Check sheet for the modelled part. Datum: model origin and axes. Units: mm. A direction names the side the tool comes from. Round coordinates to 2 decimals unless told otherwise and drop trailing zeros. Write each loop counter-clockwise with the first axis right and the second up, starting at its lowest first coordinate (ties: lowest second). Pieces come first, ordered by that corner, then holes. Notation, with made-up numbers: (-27, 54) -> (2, 54) arc R12 ccw to (2, 72) -> close; hole circle Ø8 at (46, -10.75). An arc over 180 degrees is marked (long way). One line per item, written item: value.
Autodesk Inventor part; units mm, degrees
ref_plane "YZ Plane" through (0, 0, 0) normal (1, 0, 0) x (0, 1, 0)
ref_plane "XZ Plane" through (0, 0, 0) normal (0, 1, 0) x (-1, 0, 0)
ref_plane "XY Plane" through (0, 0, 0) normal (0, 0, 1) x (1, 0, 0)
sketch "Sketch1" plane through (0, 0, 0) normal (0, 1, 0) x (-1, 0, 0)
  line L0 (-19.05, -25.4) -> (19.05, -25.4)
  line L1 (19.05, -25.4) -> (19.05, 25.4)
  line L2 (19.05, 25.4) -> (-19.05, 25.4)
  line L3 (-19.05, 25.4) -> (-19.05, -25.4)
  line L4 (-19.05, -25.4) -> (19.05, 25.4) construction
  line L5 (19.05, -25.4) -> (-19.05, 25.4) construction
  line L6 (-15.875, 22.225) -> (15.875, 22.225)
  line L7 (15.875, 22.225) -> (15.875, -22.225)
  line L8 (15.875, -22.225) -> (-15.875, -22.225)
  line L9 (-15.875, -22.225) -> (-15.875, 22.225)
  point P0 (0, 0)
  dimension "d0" = 38.1
  dimension "d1" = 50.8
  dimension "d2" = 3.175
extrude "Extrusion1" add sketch "Sketch1" along normal blind 508
sketch "Sketch2" plane through (19.05, 0, 25.4) normal (1, 0, 0) x (0, 0, -1)
  line L0 (25.4, 469.9) -> (25.4, 393.7) construction
  line L1 (12.7, 469.9) -> (12.7, 393.7)
  line L2 (38.1, 393.7) -> (38.1, 469.9)
  arc A0 (38.1, 469.9) -> (12.7, 469.9) centre (25.4, 469.9) ccw
  arc A1 (12.7, 393.7) -> (38.1, 393.7) centre (25.4, 393.7) ccw
  line L3 (25.4, 298.45) -> (25.4, 146.05) construction
  line L4 (12.7, 298.45) -> (12.7, 146.05)
  line L5 (38.1, 146.05) -> (38.1, 298.45)
  arc A2 (38.1, 298.45) -> (12.7, 298.45) centre (25.4, 298.45) ccw
  arc A3 (12.7, 146.05) -> (38.1, 146.05) centre (25.4, 146.05) ccw
  line L6 (25.4, 114.3) -> (25.4, 38.1) construction
  line L7 (12.7, 114.3) -> (12.7, 38.1)
  line L8 (38.1, 38.1) -> (38.1, 114.3) construction
  arc A4 (38.1, 114.3) -> (12.7, 114.3) centre (25.4, 114.3) ccw
  arc A5 (12.7, 38.1) -> (38.1, 38.1) centre (25.4, 38.1) ccw construction
  line L9 (0, 0) -> (50.8, 0)
  line L10 (50.8, 0) -> (50.8, 508)
  line L11 (0, 508) -> (50.8, 508)
  line L12 (0, 0) -> (0, 508)
  line L13 (0, 0) -> (0, 508)
  circle A6 centre (25.4, 346.075) radius 12.7
  circle A7 centre (25.4, 25.4) radius 25.4
  circle A8 centre (25.4, 25.4) radius 14.2875
  circle A9 centre (25.4, 222.25) radius 12.7
  arc A10 (12.7, 247.65) -> (38.1, 247.65) centre (25.4, 247.65) ccw
  arc A11 (38.1, 196.85) -> (12.7, 196.85) centre (25.4, 196.85) ccw
  point P0 (25.4, 0)
  point P1 (25.4, 431.8)
  point P2 (25.4, 76.2)
  point P3 (25.4, 0)
  point P4 (25.4, 0)
  point P5 (0, 25.4)
  point P6 (50.8, 25.4)
  dimension "d5" = 25.4
  dimension "d6" = 25.4
  dimension "d7" = 25.4
  dimension "d8" = 508
  dimension "d9" = 76.2
  dimension "d10" = 152.4
  dimension "d11" = 76.2
  dimension "d15" = 25.4
  dimension "d16" = 161.925
  dimension "d18" = 38.1
  dimension "d19" = 38.1
  dimension "d35" = 28.575
  dimension "d49" = 298.45
  dimension "d52" = 25.4
extrude "Extrusion2" cut sketch "Sketch2" against normal blind 508 contours A0 L2 A1 L1 | A2 L5 A10 L4 | A11 L5 A3 L4 | L12 A7 L9 | A7 L10 L9 | A6 | A8
sketch "Sketch3" plane through (-19.05, 0, 25.4) normal (0, 0, 1) x (1, 0, 0)
  line L0 (19.05, 0) -> (19.05, 50.8) construction
  line L1 (19.05, 50.8) -> (19.05, 508) construction
  circle A0 centre (19.05, 101.6) radius 2.4892
  circle A1 centre (19.05, 177.8) radius 2.4892
  circle A2 centre (19.05, 254) radius 2.4892
  circle A3 centre (19.05, 330.2) radius 2.4892
  circle A4 centre (19.05, 406.4) radius 2.4892
  circle A5 centre (19.05, 482.6) radius 2.4892
  dimension "d20" = 50.8
  dimension "d21" = 457.2
  dimension "d22" = 4.9784
  dimension "d23" = 50.8
  dimension "d26" = 76.2
extrude "Extrusion3" cut sketch "Sketch3" against normal blind 25.4
sketch "Sketch5" plane through (-15.875, 508, 22.225) normal (1, 0, 0) x (0, 0, -1)
  circle A0 centre (22.225, -482.6) radius 14.2875
  circle A1 centre (22.225, -482.6) radius 26.9875
  point P0 (22.225, -508)
  dimension "d36" = 53.975
extrude "Extrusion5" cut sketch "Sketch5" along normal up to surface (31.75 mm away)
sketch "Sketch6" plane through (19.05, 508, 25.4) normal (1, 0, 0) x (0, 0, -1)
  circle A0 centre (25.4, -411.5562) radius 9.6012
  circle A1 centre (25.4, -411.5562) radius 25.4 construction
  line L0 (15.6798, -388.0897) -> (35.1202, -388.0897) construction
  line L1 (35.1202, -388.0897) -> (35.1202, -435.0227) construction
  line L2 (35.1202, -435.0227) -> (15.6798, -435.0227) construction
  line L3 (15.6798, -435.0227) -> (15.6798, -388.0897) construction
  arc A2 (0, -482.6) -> (50.8, -482.6) centre (25.4, -482.6) ccw
  circle A3 centre (15.6798, -388.0897) radius 2.4892
  circle A4 centre (1.9335, -401.836) radius 2.4892 construction
  circle A5 centre (1.9335, -421.2764) radius 2.4892 construction
  circle A6 centre (15.6798, -435.0227) radius 2.4892
  circle A7 centre (35.1202, -435.0227) radius 2.4892
  circle A8 centre (48.8665, -421.2764) radius 2.4892 construction
  circle A9 centre (48.8665, -401.836) radius 2.4892 construction
  circle A10 centre (35.1202, -388.0897) radius 2.4892
  point P0 (25.4, -508)
  point P1 (25.4, -508)
  dimension "d39" = 19.2024
  dimension "d40" = 50.8
  dimension "d41" = 4.9784
  dimension "d44" = 360
  dimension "d46" = 71.0438
extrude "Extrusion6" cut sketch "Sketch6" against normal blind 25.4
sketch "Sketch8" plane through (-19.05, 508, -25.4) normal (-1, 0, 0) x (0, 0, 1)
  circle A0 centre (25.4, -411.5562) radius 9.6012
  circle A1 centre (25.4, -411.5562) radius 15.875
  point P0 (25.4, -508)
  dimension "d53" = 31.75
extrude "Extrusion7" cut sketch "Sketch8" against normal blind 25.4 contours A0 | A1
sketch "Sketch9" plane through (19.05, 508, -25.4) normal (0, 0, -1) x (-1, 0, 0)
  line L0 (34.925, -467.2907) -> (3.175, -467.2907)
  line L1 (3.175, -467.2907) -> (3.175, -473.4805)
  line L2 (34.925, -467.2907) -> (34.925, -473.4805)
  line L3 (3.175, -473.4805) -> (34.925, -473.4805)
  line L4 (3.175, -467.2907) -> (3.175, -463.4807)
  line L5 (3.175, -467.2907) -> (3.175, 0)
  line L6 (3.175, -463.4807) -> (34.925, -463.4807)
  line L7 (34.925, -467.2907) -> (34.925, 0)
  point P0 (19.05, -508)
  dimension "d64" = 3.81
extrude "Extrusion8" cut sketch "Sketch9" against normal through all
sketch "Sketch10" plane through (19.05, 508, 25.4) normal (1, 0, 0) x (0, 0, -1)
  circle A0 centre (25.4, -482.6) radius 14.2875
  circle A1 centre (25.4, -482.6) radius 22.225
  line L0 (50.8, -482.6) -> (50.8, 0)
  arc A2 (25.4, -504.825) -> (50.8, -479.425) centre (25.4, -479.425) ccw
  line L1 (0, -482.6) -> (0, 0)
  arc A3 (0, -479.425) -> (25.4, -504.825) centre (25.4, -479.425) ccw
  arc A4 (0, -482.6) -> (50.8, -482.6) centre (25.4, -482.6) ccw
  point P0 (25.4, -508)
  point P1 (25.4, -504.825)
  dimension "d58" = 44.45
extrude "Extrusion9" [suppressed]
chamfer "Chamfer1" distance 3.175 angle 45 2 edges at (0, 44.5193, -22.225) (0, 44.5193, 22.225)
sketch "Sketch11" plane through (19.05, 508, -25.4) normal (0, 0, -1) x (-1, 0, 0)
  circle A0 centre (19.05, -25.4) radius 2.4892 construction
  circle A1 centre (19.05, -25.4) radius 1.5875
  line L0 (34.925, -463.4807) -> (34.925, -482.6)
  line L1 (38.1, -482.6) -> (34.925, -482.6)
  line L2 (38.1, -482.6) -> (38.1, 0)
  line L3 (0, 0) -> (38.1, 0)
  line L4 (0, -482.6) -> (0, 0)
  line L5 (3.175, -482.6) -> (0, -482.6)
  line L6 (3.175, -482.6) -> (3.175, -463.4807)
  line L7 (3.175, -463.4807) -> (34.925, -463.4807)
  circle A2 centre (19.05, -101.6) radius 1.5875
  circle A3 centre (19.05, -177.8) radius 1.5875
  circle A4 centre (19.05, -254) radius 1.5875
  circle A5 centre (19.05, -330.2) radius 1.5875
  circle A6 centre (19.05, -406.4) radius 1.5875
  point P0 (19.05, -508)
  dimension "d65" = 3.175
  dimension "d68" = 76.2
extrude "Extrusion10" cut sketch "Sketch11" against normal blind 25.4 contours A1 | A2 | A3 | A4 | A5 | A6
thread "Thread1"
thread "Thread2"
thread "Thread3"
thread "Thread4"
thread "Thread5"
thread "Thread6"
properties part number "CLIM_002_ClimbPole" material "Aluminum 6061"
Item 1: Thickness scan on line 1 (X direction, y = 249.5, z = -14.5) (3 decimals); line 2 (Z direction, x = -4.5, y = 345.5) (3 decimals); line 3 (Z direction, x = -16.65, y = 25.4). Record the ranges inside material, lowest first.
Answer:
line 1: x = -19.05 to -15.875, 15.875 to 19.05
line 2: z = -25.4 to -22.225, 22.225 to 25.4
line 3: z = -25.4 to -14.29, 14.29 to 25.4
Item 2: Depth check by flat-ended pin: P1, Ø3.5, axis at x = 0, y = 177.8, coming from the +Z side (3 decimals); P2, Ø4, axis at y = 119.91, z = 9.72, coming from the +X side (3 decimals); P3, Ø12, axis at x = -2, z = -19.5, coming from the -Y side. Enter the tip coordinate at first touch or a pass-through.
Answer:
P1: stops at z = -22.225
P2: stops at x = -15.875
P3: stops at y = 44.52
Item 3: Tool access check on faces 1 (the flat face through (0, 275, 22.225)), 2 (the cylindrical face through (-17.44, 482.597, -0.279)), 3 (the flat face through (17, 508, 0)). Record the directions out of +Z, -Z, +X, -X, +Y, -Y that give a thin tool (end or side, any length) a straight path to the whole face; none if there is none.
Answer:
face 1: +Y, -Y
face 2: +X, -X
face 3: +Z, -Z, +X, -X, +Y
Item 4: Sectioned sample at B-B on y = 369. Enter the section's corners in (x, z) (3 decimals).
Answer:
outline: (-19.05, -25.4) -> (19.05, -25.4) -> (19.05, 25.4) -> (-19.05, 25.4) -> close; hole (-15.875, -22.225) -> (15.875, -22.225) -> (15.875, 22.225) -> (-15.875, 22.225) -> close
Item 5: Sectioned sample at A-A on y = 154. Enter the section's corners in (x, z) (3 decimals), and give its area (3 significant figures).
Answer:
outline: (-19.05, -25.4) -> (19.05, -25.4) -> (19.05, -12.7) -> (15.875, -12.7) -> (15.875, -22.225) -> (-15.875, -22.225) -> (-15.875, -12.7) -> (-19.05, -12.7) -> close; (-19.05, 12.7) -> (-15.875, 12.7) -> (-15.875, 22.225) -> (15.875, 22.225) -> (15.875, 12.7) -> (19.05, 12.7) -> (19.05, 25.4) -> (-19.05, 25.4) -> close
area: 363 mm^2
Item 6: Sectioned sample at C-C on z = 0. Count the separate pieces of the cut face and the enclosed holes in it, and give its area (3 significant figures).
Answer:
separate pieces: 14
enclosed holes: 0
area: 1,110 mm^2
Item 7: Mould release check, pull along Z, two halves, no side actions. Record for faces 4 (the cylindrical face through (-17.485, 80.946, -3.441)), 5 (the flat face through (19.05, 250, 17)), 6 (the cylindrical face through (-17.44, 0.006, 0.559)): pulls with the +Z half, pulls with the -Z half, needs draft (parallel to the pull), parting line crosses it, or undercut.
Answer:
face 4: undercut
face 5: needs draft
face 6: parting line crosses it
